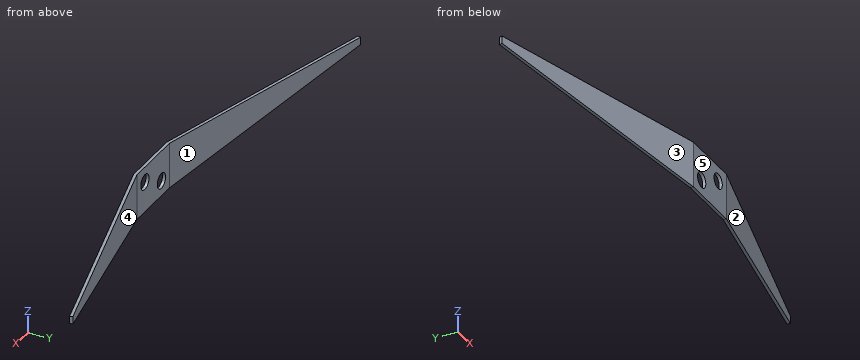
from build123d import *

# Parameters (mm, degrees)
F1_DEPTH = 15
F3_DEPTH = 21.672449
F5_D     = 5


with BuildPart() as f1:
    # F0 (on Top) → F1 (new body)
    with BuildSketch(Plane.XY):
        Polygon((-77.274066, 20.705524), (0, 0), (20, 0), (97.274066, 20.705524), (97.015247, 21.671449), (19.868348, 1), (0.131652, 1), (-77.015247, 21.671449), align=None)
    extrude(amount=F1_DEPTH)

    # F2 (on Front) → F3 (cut, through all)
    with BuildSketch(Plane.XZ):
        Polygon((-80, 0), (0, 0), (-80, 13), align=None)
        Polygon((99.983092, 13), (19.983092, 0), (99.983092, 0), align=None)
    extrude(amount=-F3_DEPTH, mode=Mode.SUBTRACT)

    # F5 (through all)
    with Locations(Plane.XZ):
        with Locations((5, 5), (15, 10)):
            Hole(F5_D / 2)


solid = f1.part
Source: CAD feature listing. Evaluate the final solid. Frame: model axes, mm. Face numbers are marked on the shaded views. A direction names the side the tool comes from. Round coordinates to 2 decimals unless told otherwise and drop trailing zeros. Loops run counter-clockwise (first coordinate to the right, second up) from the corner with the lowest first, then second, coordinate; pieces in that order, holes last. Notation, with made-up numbers: M 80.25,14 L 138.25,14 A7 ccw 138.25,19 Z; hole C -19,56.25 d2. An arc over 180 degrees is marked long. Return JSON: item names as keys, results as strings. Group by question number.
1. Reachability of the marked faces 4 and 5 from +Z, -Z, +X, -X, +Y, -Y: full face, straight path, thin tool, end or side. Return the list, or none.
2. Section query D-D on x = 68. Output: boundary loops of the cut face in (y, z).
3. Mould query, pull axis X, two halves, no side actions, for the marked faces 1, 2 and 3. Classes: released by +X, released by -X, zero draft, split by the parting line, or undercut.
4. Section query A-A on x = 5. Output: boundary loops of the cut face in (y, z), and give its area (3 significant figures).
5. Section query B-B on y = 6.25. Output: boundary loops of the cut face in (x, z), and give its area (3 significant figures).
6. Section query C-C on z = 10. Output: boundary loops of the cut face in (x, y).
7. Material intervals for line 1 along Z through (x, y) = (5, 0.4); line 2 along Y through (x, z) = (14, 2.5); line 3 along Y through (x, z) = (73.5, 13), sorted ascending. Write a range as from..to.
8. Pin query (flat end, axial travel): pin 1 (10 mm diameter, centred on x = -38.5, y = 12.5, fed in from -Z); pin 2 (7.5 mm diameter, centred on x = 10, z = 7, fed in from +Y). Return the tip coordinate at first contact, or that it passes through.
Checks:
{
 "1": {"face 4": "+Z, -Z, +Y", "face 5": "+Z, -Z, +X, -X, -Y"},
 "2": {"outline": "M 12.86,7.8 L 13.9,7.8 L 13.9,15 L 12.86,15 Z"},
 "3": {"face 1": "undercut", "face 2": "released by +X", "face 3": "released by -X"},
 "4": {"outline": "M 0,0 L 1,0 L 1,2.5 L 0,2.5 Z; M 0,7.5 L 1,7.5 L 1,15 L 0,15 Z", "area": "10.0 mm²"},
 "5": {"outline": "M -23.33,3.79 L -19.46,3.16 L -19.46,15 L -23.33,15 Z; M 39.46,3.17 L 43.33,3.79 L 43.33,15 L 39.46,15 Z", "area": "89.0 mm²"},
 "6": {"outline": "M -61.54,16.49 L 0,0 L 12.5,0 L 12.5,1 L 0.13,1 L -61.54,17.52 Z; M 17.5,0 L 20,0 L 81.52,16.48 L 81.52,17.52 L 19.87,1 L 17.5,1 Z"},
 "7": {"line 1": "z = 0..2.5, 7.5..15", "line 2": "y = 0..1", "line 3": "y = 14.34..15.37"},
 "8": {"pin 1": "stops at z = 5.54", "pin 2": "stops at y = 1"}
}
